Autodesk Fusion 360 part; units mm, degrees
sketch "Sketch1" plane through (0, 0, 0) normal (0, 0, 1) x (1, 0, 0)
  line L0 (-7, 1.5) -> (35, 1.5)
  line L1 (35, 1.5) -> (35, -3.5)
  line L2 (35, -3.5) -> (-7, -3.5)
  line L3 (-7, -3.5) -> (-7, 1.5)
  line L4 (-7, 1.5) -> (-7, 10)
  line L5 (-7, 10) -> (-2, 4.3)
  line L6 (-2, 4.3) -> (-2, 1.5)
  line L7 (35, 1.5) -> (35, 10)
  line L8 (35, 10) -> (30, 4.3)
  line L9 (30, 4.3) -> (30, 1.5)
  dimension "d1" = 5
  dimension "d2" = 42
  dimension "d13" = 8.5
  dimension "d14" = 5
  dimension "d15" = 2.8
extrude "Extrude1" add sketch "Sketch1" along normal blind 3
sketch "Sketch2" plane through (0, 0, 3) normal (0, 0, 1) x (-1, 0, 0)
  line L0 (-35, 3.5) -> (-35, -10)
  line L1 (-35, -10) -> (-30, -4.3)
  line L2 (-30, -4.3) -> (-30, -1.5)
  line L3 (-30, -1.5) -> (2, -1.5)
  line L4 (2, -1.5) -> (2, -4.3)
  line L5 (2, -4.3) -> (7, -10)
  line L6 (7, -10) -> (7, 3.5)
  line L7 (7, 3.5) -> (-35, 3.5)
  line L8 (-7, -1.5) -> (-21, -1.5)
  line L9 (-21, -1.5) -> (-21, 3.5)
  line L10 (-21, 3.5) -> (-7, 3.5)
  line L11 (-7, 3.5) -> (-7, -1.5)
  line L12 (-7, -1.5) -> (-21, 3.5) construction
  line L13 (-21, -1.5) -> (-7, 3.5) construction
  point P0 (-14, 1)
  dimension "d16" = 14
  dimension "d17" = 14
  dimension "d18" = 5
extrude "Extrude2" cut sketch "Sketch2" against normal blind 1 contours L3 L7 L8 L9 L10 L11
sketch "Sketch3" plane through (0, 0, 3) normal (0, 0, 1) x (-1, 0, 0)
  line L0 (-21, -1.5) -> (-21, 3.5)
  line L1 (-21, 3.5) -> (-35, 3.5)
  line L2 (-35, 3.5) -> (-35, -10)
  line L3 (-35, -10) -> (-30, -4.3)
  line L4 (-30, -4.3) -> (-30, -1.5)
  line L5 (-30, -1.5) -> (-21, -1.5)
  line L6 (6, -1.5) -> (-34, -1.5)
  line L7 (-34, -1.5) -> (-34, 3.5)
  line L8 (-34, 3.5) -> (6, 3.5)
  line L9 (6, 3.5) -> (6, -1.5)
  line L10 (6, -1.5) -> (-34, 3.5) construction
  line L11 (-34, -1.5) -> (6, 3.5) construction
  ellipse E0 centre (3.25, 1) end of major axis (4.5, 1) minor radius 2
  line L12 (2, 1) -> (4.5, 1) construction
  line L13 (3.25, -1) -> (3.25, 3) construction
  line L14 (3.2507, 3.5) -> (3.25, 3)
  line L15 (3.25, -1) -> (3.25, -1.5)
  ellipse E1 centre (-31.25, 0.9902) end of major axis (-32.5, 0.9902) minor radius 2
  line L16 (-30, 0.9902) -> (-32.5, 0.9902) construction
  line L17 (-31.25, 2.9902) -> (-31.25, -1.0098) construction
  line L18 (-31.25, 2.9902) -> (-31.25, 3.5)
  line L19 (-31.25, -1.5) -> (-31.25, -1.0098)
  line L20 (6, -2.5) -> (2, -2.5)
  line L21 (2, -2.5) -> (2, -1.5)
  line L22 (2, -1.5) -> (6, -1.5)
  line L23 (6, -1.5) -> (6, -2.5)
  line L24 (-34, -1.5) -> (-30, -1.5)
  line L25 (-30, -1.5) -> (-30, -2.5)
  line L26 (-30, -2.5) -> (-34, -2.5)
  line L27 (-34, -2.5) -> (-34, -1.5)
  point P0 (-14, 1)
  dimension "d7" = 40
  dimension "d8" = 2.5
  dimension "d9" = 4
  dimension "d10" = 2.5
  dimension "d19" = 5
  dimension "d20" = 21
  dimension "d21" = 2.5
  dimension "d22" = 37
  dimension "d23" = 1.5
  dimension "d24" = 5
extrude "Extrude3" add sketch "Sketch3" along normal blind 3 contours L4 L6 L24 L25 L26 L27 | L6 L20 L21 L22 L23 | L1 L6 L7 L8 E1 L18 L19 L24 | L6 L8 L9 E0 L14 L15 L22
sketch "Sketch6" plane through (0, -3.5, 0) normal (0, -1, 0) x (1, 0, 0)
  line L0 (21, 3) -> (21, 2)
  line L1 (21, 2) -> (7, 2)
  line L2 (7, 2) -> (7, 3)
  line L3 (7, 3) -> (-3.2507, 3)
  line L4 (-3.2507, 3) -> (-3.2507, 6)
  line L5 (-3.2507, 6) -> (-6, 6)
  line L6 (-6, 6) -> (-6, 3)
  line L7 (-6, 3) -> (-7, 3)
  line L8 (-7, 3) -> (-7, 0)
  line L9 (-7, 0) -> (35, 0)
  line L10 (35, 0) -> (35, 3)
  line L11 (35, 3) -> (34, 3)
  line L12 (34, 3) -> (34, 6)
  line L13 (34, 6) -> (31.25, 6)
  line L14 (31.25, 6) -> (31.25, 3)
  line L15 (31.25, 3) -> (21, 3)
  line L16 (-2, 6) -> (-6, 6)
  line L17 (-6, 6) -> (-6, 0)
  line L18 (-6, 0) -> (-2, 0)
  line L19 (-2, 0) -> (-2, 6)
  line L20 (34, 6) -> (30, 6)
  line L21 (30, 6) -> (30, 0)
  line L22 (30, 0) -> (34, 0)
  line L23 (34, 0) -> (34, 6)
extrude "Extrude6" add sketch "Sketch6" along normal blind 1 contours L14 L15 L20 L21 | L9 L12 L13 L14 L15 L20 L21 L22 L23 | L3 L4 L5 L6 L9 L16 L17 L18 L19 | L3 L4 L16 L19
sketch "Sketch4" plane through (0, 0, 0) normal (0, 0, -1) x (1, 0, 0)
  line L0 (35, -10) -> (35, 3.5)
  line L1 (35, 3.5) -> (34, 3.5)
  line L2 (-7, 3.5) -> (-7, -10)
  line L3 (-7, -10) -> (-2, -4.3)
  line L4 (-2, -4.3) -> (-2, -1.5)
  line L5 (-2, -1.5) -> (30, -1.5)
  line L6 (30, -1.5) -> (30, -4.3)
  line L7 (30, -4.3) -> (35, -10)
  line L8 (5, 3.5) -> (23, 3.5)
  line L9 (23, 3.5) -> (23, -1.5)
  line L10 (23, -1.5) -> (5, -1.5)
  line L11 (5, -1.5) -> (5, 3.5)
  circle A0 centre (14, 1) radius 1.125
  line L12 (34, 3.5) -> (34, 4.5)
  line L13 (34, 4.5) -> (30, 4.5)
  line L14 (30, 4.5) -> (30, 3.5)
  line L15 (30, 3.5) -> (-2, 3.5)
  line L16 (-2, 3.5) -> (-2, 4.5)
  line L17 (-2, 4.5) -> (-6, 4.5)
  line L18 (-6, 4.5) -> (-6, 3.5)
  line L19 (-6, 3.5) -> (-7, 3.5)
  dimension "d25" = 2.25
extrude "Extrude4" cut sketch "Sketch4" against normal blind 2 contours A0
sketch "Sketch5" plane through (0, 0, 0) normal (0, 0, -1) x (1, 0, 0)
  circle A0 centre (14, 1) radius 1.125
  line L0 (35, -10) -> (35, 3.5)
  line L1 (35, 3.5) -> (34, 3.5)
  line L2 (-7, 3.5) -> (-7, -10)
  line L3 (-7, -10) -> (-2, -4.3)
  line L4 (-2, -4.3) -> (-2, -1.5)
  line L5 (-2, -1.5) -> (30, -1.5)
  line L6 (30, -1.5) -> (30, -4.3)
  line L7 (30, -4.3) -> (35, -10)
  circle A1 centre (14, 1) radius 1.875
  line L8 (34, 3.5) -> (34, 4.5)
  line L9 (34, 4.5) -> (30, 4.5)
  line L10 (30, 4.5) -> (30, 3.5)
  line L11 (30, 3.5) -> (-2, 3.5)
  line L12 (-2, 3.5) -> (-2, 4.5)
  line L13 (-2, 4.5) -> (-6, 4.5)
  line L14 (-6, 4.5) -> (-6, 3.5)
  line L15 (-6, 3.5) -> (-7, 3.5)
  dimension "d28" = 3.75
extrude "Extrude5" cut sketch "Sketch5" against normal blind 1.25 contours A1
equation "d16 = d17"
equation "d18 = d1"
equation "d19 = d1"
equation "d20 = d2 / 2"
equation "d21 = d1 / 2"
equation "d24 = d1"
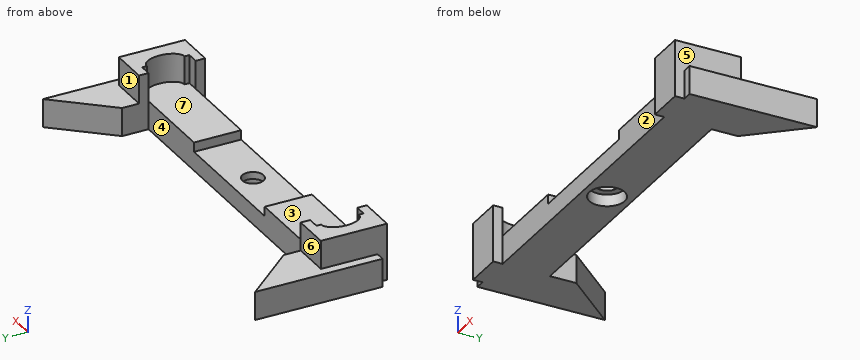
Geometry: final body of the model. Coordinates: model frame, mm. Face numbers are marked on the shaded views. A direction names the side the tool comes from. Give positions to 0.01 mm unless a question says otherwise; leave off trailing zeros. Loops run counter-clockwise (first coordinate to the right, second up) from the corner with the lowest first, then second, coordinate; pieces in that order, holes last. Notation, with made-up numbers: M 34,56.25 L 43,56.25 A8 ccw 43,62.25 Z; hole C 33,70.5 d10. An arc over 180 degrees is marked long. Put each result on its own line as item: value.
1) Mould query, pull axis Y, two halves, no side actions, for the marked faces 5, 6 and 7. Classes: released by +Y, released by -Y, zero draft, split by the parting line, or undercut.
Computed values:
face 5: zero draft
face 6: released by +Y
face 7: undercut
2) Cut plane C-C, the plane y = 4.75. Return the cut outline in (x, z), plus the area to 3 significant figures.
Computed values:
outline: M -7,0 L -2.39,0 L -2.39,3 L -7,3 Z; M 30.39,0 L 35,0 L 35,3 L 30.39,3 Z
area: 27.6 mm^2
3) Cut plane D-D, the plane x = 20.5. Return the cut outline in (y, z), plus the area to 3 significant figures.
Computed values:
outline: M -3.5,0 L 1.5,0 L 1.5,2 L -3.5,2 Z
area: 10.0 mm^2
4) Material intervals for L1, parallel to Y at x = 14, z = 0.3 (3 decimals); L2, parallel to X at y = -1, z = 1.8 (3 decimals); L3, parallel to X at y = 0, z = 2.35, sorted ascending. Write a range as from..to.
Computed values:
L1: y = -3.5..-2.875, 0.875..1.5
L2: x = -7..12.875, 15.125..35
L3: x = -7..7, 21..35
5) Cut plane A-A, the plane x = 14. Return the cut outline in (y, z) (3 decimals), plus the area to 4 significant figures.
Computed values:
outline: M -3.5,0 L -2.875,0 L -2.875,1.25 L -2.125,1.25 L -2.125,2 L -3.5,2 Z; M 0.125,1.25 L 0.875,1.25 L 0.875,0 L 1.5,0 L 1.5,2 L 0.125,2 Z
area: 3.625 mm^2
6) Reachability of the marked faces 1, 2, 3 and 4 from +Z, -Z, +X, -X, +Y, -Y: full face, straight path, thin tool, end or side. Return the list, or none.
Computed values:
face 1: +Z, +X, -X, +Y
face 2: +Z, -Z, -Y
face 3: +Z
face 4: +Z, -Z, +Y
7) Cut plane B-B, the plane z = 0.6. Return the cut outline in (x, y) (3 decimals), plus the area to 3 significant figures.
Computed values:
outline: M -7,-3.5 L -6,-3.5 L -6,-4.5 L -2,-4.5 L -2,-3.5 L 30,-3.5 L 30,-4.5 L 34,-4.5 L 34,-3.5 L 35,-3.5 L 35,10 L 30,4.3 L 30,1.5 L -2,1.5 L -2,4.3 L -7,10 Z; hole C 14,-1 d3.75
area: 263 mm^2
8) First-contact query: P1, Ø4, axis at x = 27, y = -1.5, coming from the +Z side; P2, Ø3, axis at x = 25, z = 3.5, coming from the +Y side; P3, Ø1.5, axis at y = -2, z = 5, coming from the -X side. Flat tips, straight axial feed; report the tip coordinate or a pass-through.
Computed values:
P1: stops at z = 3
P2: stops at y = 1.5
P3: stops at x = -6
